from build123d import *

# Parameters (mm, degrees)
SKETCH1_R           = 0.775
SKETCH1_W           = 2
SKETCH1_H           = 3.5
SKETCH1_W_2         = 2.5
SKETCH1_H_2         = 6.5
BOSS_EXTRUDE1_DEPTH = 2
SKETCH2_R           = 1.275
CUT_EXTRUDE1_DEPTH  = 0.5
SKETCH3_W           = 8
SKETCH3_H           = 11
CUT_EXTRUDE2_DEPTH  = 3


with BuildPart() as part:
    # Sketch1 → Boss-Extrude1 (new body)
    with BuildSketch(Plane(origin=(0, 0, 0), x_dir=(1, 0, 0), z_dir=(0, 1, 0))):
        with BuildLine():
            Line((-0.26263299, 9.170981105), (-0.26263299, -1.829018895))
            Line((-0.26263299, -1.829018895), (-7.76263299, -1.829018895))
            Line((-7.76263299, -1.829018895), (-7.76263299, 9.170981105))
            Line((-7.76263299, 9.170981105), (-19.76263299, 9.170981105))
            Line((-19.76263299, 9.170981105), (-19.76263299, -1.829018895))
            Line((-19.76263299, -1.829018895), (-27.26263299, -1.829018895))
            Line((-27.26263299, -1.829018895), (-27.26263299, 9.170981105))
            Line((-27.26263299, 9.170981105), (-34.51263299, 9.170981105))
            Line((-34.51263299, 9.170981105), (-35.51263299, 9.170981105))
            ThreePointArc((-35.51263299, 9.170981105), (-38.341060114, 7.99940823), (-39.51263299, 5.170981105))
            Line((-39.51263299, 5.170981105), (-39.51263299, -22.829018895))
            ThreePointArc((-39.51263299, -22.829018895), (-38.341060114, -25.65744602), (-35.51263299, -26.829018895))
            Line((-35.51263299, -26.829018895), (-34.51263299, -26.829018895))
            Line((-34.51263299, -26.829018895), (65.48736701, -26.829018895))
            Line((65.48736701, -26.829018895), (66.48736701, -26.829018895))
            ThreePointArc((66.48736701, -26.829018895), (69.315794135, -25.65744602), (70.48736701, -22.829018895))
            Line((70.48736701, -22.829018895), (70.48736701, 5.170981105))
            ThreePointArc((70.48736701, 5.170981105), (69.315794135, 7.99940823), (66.48736701, 9.170981105))
            Line((66.48736701, 9.170981105), (65.48736701, 9.170981105))
            Line((65.48736701, 9.170981105), (58.23736701, 9.170981105))
            Line((58.23736701, 9.170981105), (58.23736701, -1.829018895))
            Line((58.23736701, -1.829018895), (50.73736701, -1.829018895))
            Line((50.73736701, -1.829018895), (50.73736701, 9.170981105))
            Line((50.73736701, 9.170981105), (38.73736701, 9.170981105))
            Line((38.73736701, 9.170981105), (38.73736701, -1.829018895))
            Line((38.73736701, -1.829018895), (31.23736701, -1.829018895))
            Line((31.23736701, -1.829018895), (31.23736701, 9.170981105))
            Line((31.23736701, 9.170981105), (19.23736701, 9.170981105))
            Line((19.23736701, 9.170981105), (19.23736701, -1.829018895))
            Line((19.23736701, -1.829018895), (11.73736701, -1.829018895))
            Line((11.73736701, -1.829018895), (11.73736701, 9.170981105))
            Line((11.73736701, 9.170981105), (-0.26263299, 9.170981105))
        make_face()
        with Locations((-37.01263299, 4.170981105)):
            Circle(SKETCH1_R, mode=Mode.SUBTRACT)
        with Locations((-37.01263299, -21.829018895)):
            Circle(SKETCH1_R, mode=Mode.SUBTRACT)
        with Locations((67.98736701, 4.170981105)):
            Circle(SKETCH1_R, mode=Mode.SUBTRACT)
        with Locations((67.98736701, -21.829018895)):
            Circle(SKETCH1_R, mode=Mode.SUBTRACT)
        with Locations((-24.16263299, -4.379018895)):
            Rectangle(SKETCH1_W, SKETCH1_H, mode=Mode.SUBTRACT)
        with Locations((-4.66263299, -4.379018895)):
            Rectangle(SKETCH1_W, SKETCH1_H, mode=Mode.SUBTRACT)
        with Locations((14.83736701, -4.379018895)):
            Rectangle(SKETCH1_W, SKETCH1_H, mode=Mode.SUBTRACT)
        with Locations((34.33736701, -4.379018895)):
            Rectangle(SKETCH1_W, SKETCH1_H, mode=Mode.SUBTRACT)
        with Locations((53.83736701, -4.379018895)):
            Rectangle(SKETCH1_W, SKETCH1_H, mode=Mode.SUBTRACT)
        with Locations((-9.21263299, -18.479018895)):
            Rectangle(SKETCH1_W_2, SKETCH1_H_2, mode=Mode.SUBTRACT)
        with Locations((-28.71263299, -18.479018895)):
            Rectangle(SKETCH1_W_2, SKETCH1_H_2, mode=Mode.SUBTRACT)
        with Locations((10.28736701, -18.479018895)):
            Rectangle(SKETCH1_W_2, SKETCH1_H_2, mode=Mode.SUBTRACT)
        with Locations((29.78736701, -18.479018895)):
            Rectangle(SKETCH1_W_2, SKETCH1_H_2, mode=Mode.SUBTRACT)
        with Locations((49.28736701, -18.479018895)):
            Rectangle(SKETCH1_W_2, SKETCH1_H_2, mode=Mode.SUBTRACT)
    extrude(amount=BOSS_EXTRUDE1_DEPTH)

    # Sketch2 → Cut-Extrude1 (cut)
    with BuildSketch(Plane(origin=(0, 2, 0), x_dir=(1, 0, 0), z_dir=(0, 1, 0))):
        with Locations((-37.01263299, 4.170981105)):
            Circle(SKETCH2_R)
        with Locations((-37.01263299, -21.829018895)):
            Circle(SKETCH2_R)
        with Locations((67.98736701, 4.170981105)):
            Circle(SKETCH2_R)
        with Locations((67.98736701, -21.829018895)):
            Circle(SKETCH2_R)
    extrude(amount=-CUT_EXTRUDE1_DEPTH, mode=Mode.SUBTRACT)

    # Sketch3 → Cut-Extrude2 (cut, through all)
    with BuildSketch(Plane(origin=(0, 2, 0), x_dir=(1, 0, 0), z_dir=(0, 1, 0))):
        with Locations((-23.51263299, 3.670981105)):
            Rectangle(SKETCH3_W, SKETCH3_H)
        with Locations((-4.01263299, 3.670981105)):
            Rectangle(SKETCH3_W, SKETCH3_H)
        with Locations((15.48736701, 3.670981105)):
            Rectangle(SKETCH3_W, SKETCH3_H)
        with Locations((34.98736701, 3.670981105)):
            Rectangle(SKETCH3_W, SKETCH3_H)
        with Locations((54.48736701, 3.670981105)):
            Rectangle(SKETCH3_W, SKETCH3_H)
    extrude(amount=-CUT_EXTRUDE2_DEPTH, mode=Mode.SUBTRACT)


solid = part.part
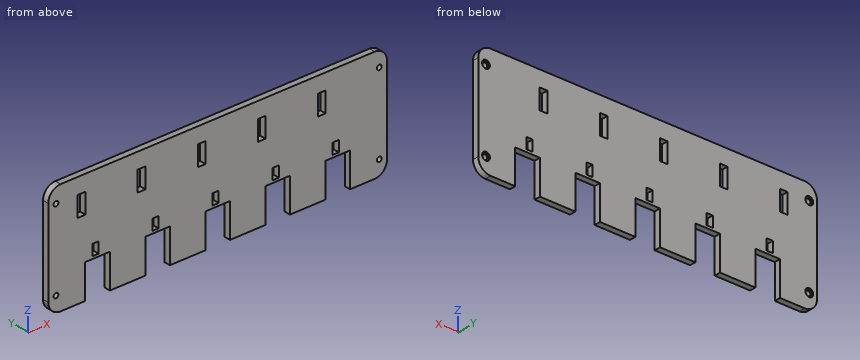
Read the model definition and answer for the solid it produces. Units are mm, in the model's axes. Give positions to 0.01 mm unless a question says otherwise; leave off trailing zeros. Loops run counter-clockwise (first coordinate to the right, second up) from the corner with the lowest first, then second, coordinate; pieces in that order, holes last. Notation, with made-up numbers: (30, 57) -> (82, 57) arc R20 ccw to (82, 88) -> close; hole circle Ø4 at (-32, 17). An arc over 180 degrees is marked (long way). Use a Markdown table: item, result.
Q1. Section A-A, the plane z = 19.5 is taken. Determine the outline of the cut face in (x, y).
Solved:
| item | result |
|---|---|
| outline | (-39.51, 0) -> (-29.96, 0) -> (-29.96, 2) -> (-39.51, 2) -> close; (-27.46, 0) -> (-10.46, 0) -> (-10.46, 2) -> (-27.46, 2) -> close; (-7.96, 0) -> (9.04, 0) -> (9.04, 2) -> (-7.96, 2) -> close; (11.54, 0) -> (28.54, 0) -> (28.54, 2) -> (11.54, 2) -> close; (31.04, 0) -> (48.04, 0) -> (48.04, 2) -> (31.04, 2) -> close; (50.54, 0) -> (70.49, 0) -> (70.49, 2) -> (50.54, 2) -> close |
Q2. Section B-B, the plane y = 0.8 is taken. Count the separate pieces of the cut face and the enclosed holes in it, then the cut area to 3 significant figures.
Solved:
| item | result |
|---|---|
| separate pieces | 1 |
| enclosed holes | 14 |
| area | 3,380 mm^2 |
Q3. Find the intervals of material crossed by line 1 along X through (y, z) = (0.8, 18.5); line 2 along X through (y, z) = (0.6, -3); line 3 along X through (y, z) = (0.6, 22), in increasing order.
Solved:
| item | result |
|---|---|
| line 1 | x = -39.51 to -29.96, -27.46 to -10.46, -7.96 to 9.04, 11.54 to 28.54, 31.04 to 48.04, 50.54 to 70.49 |
| line 2 | x = -39.51 to -27.51, -19.51 to -8.01, -0.01 to 11.49, 19.49 to 30.99, 38.99 to 50.49, 58.49 to 70.49 |
| line 3 | x = -39.51 to -37.77, -36.26 to 67.23, 68.74 to 70.49 |
Q4. Each of these flat-tipped pins is pushed along its axis until it touches: pin 1 (0.8 mm diameter, centred on x = 68, z = 21.5, fed in from +Y); pin 2 (0.6 mm diameter, centred on x = -23.5, y = 0.5, fed in from -Z). Where does it stop, or does it pass through?
Solved:
| item | result |
|---|---|
| pin 1 | passes through |
| pin 2 | stops at z = 1.83 |
